Verification items for the finished model (mm, model axes). A direction names the side the tool comes from. Give positions to 0.01 mm unless a question says otherwise; leave off trailing zeros. Write each loop counter-clockwise with the first axis right and the second up, starting at its lowest first coordinate (ties: lowest second). Pieces come first, ordered by that corner, then holes. Notation, with made-up numbers: (-30.5, -7.75) - (7.5, -7.75) arc R23 ccw to (7.5, 5.25) - close; hole circle Ø8 at (47.5, 52.5). An arc over 180 degrees is marked (long way). Answer as a JSON object with one key per item and string values. Group by question number.
Item 1: Sectioned sample at B-B, the plane y = -47. Record the boundary of the cut face in (x, z).
Item 2: Sectioned sample at D-D, the plane x = -15.5. Record the boundary of the cut face in (y, z).
Item 3: Scan lines: line 1 along X through (y, z) = (-40.5, 19); line 2 along X through (y, z) = (12.5, 25.5); line 3 along Y through (x, z) = (-8, 12.5). Record each from-to range of solid material in increasing order. Write a range as [from, to].
Item 4: Tool access check on faces 1 (the face through (-105, -51.406, 20)), 2 (the face through (-109.732, -3, 20)), 3 (the face through (18, -56.406, 20)), 4 (the face through (-99.732, -10, 20)). Record the directions out of +Z, -Z, +X, -X, +Y, -Y that give a thin tool (end or side, any length) a straight path to the whole face; none if there is none.
Item 5: Sectioned sample at A-A, the plane y = -6. Record the boundary of the cut face in (x, z).
Item 6: Go/stop test with flat-tipped pins: pin 1 (2 mm diameter, centred on y = 3.5, z = 7, fed in from +X); pin 2 (1.5 mm diameter, centred on x = 41.5, z = 6, fed in from +Y); pin 3 (11 mm diameter, centred on x = -103.5, z = 28, fed in from -Y). Record where each tip stops, or that it passes through.
Item 7: Draft check along X on faces 5 (the face through (-33, -7, 0)), 6 (the face through (70.268, -53, 20)), 7 (the face through (-70, 33.594, 20)). Enter one of: +X half, -X half, draft (parallel to the pull), parting line (faces both ways), or undercut.
```python
from build123d import *

# Parameters (mm, degrees)
SKETCH_1_W      = 10
SKETCH_1_H      = 90
SKETCH_1_W_2    = 80
SKETCH_1_H_2    = 10
SKETCH_1_W_3    = 5
SKETCH_1_H_3    = 20
SKETCH_1_H_4    = 85
EXTRUDE_1_DEPTH = 40
FILLET_1_R      = 2.5


with BuildPart() as part:
    # 草圖1 → 填料-伸長1 (new body)
    with BuildSketch(Plane.XY):
        with Locations((-34.732391425, -11.40625)):
            Rectangle(SKETCH_1_W, SKETCH_1_H)
        Polygon((-29.732391425, -56.40625), (-39.732391425, -56.40625), (-39.732391425, -66.40625), (70.267608575, -66.40625), (70.267608575, -56.40625), (65.267608575, -56.40625), align=None)
        with Locations((-69.732391425, 38.59375)):
            Rectangle(SKETCH_1_W_2, SKETCH_1_H_2)
        with Locations((67.767608575, -46.40625)):
            Rectangle(SKETCH_1_W_3, SKETCH_1_H_3)
        with Locations((-104.732391425, -8.90625)):
            Rectangle(SKETCH_1_W, SKETCH_1_H_4)
    extrude(amount=EXTRUDE_1_DEPTH)

    # 圓角1
    fillet_1_edges = [part.edges().sort_by_distance(p)[0] for p in [
        (70.267608575, -36.40625, 20),
        (65.267608575, -36.40625, 20),
    ]]
    fillet(fillet_1_edges, radius=FILLET_1_R - 0.0001)  # a hair under: the kernel refuses the full size


solid = part.part
```
Geometry check:
{
 "1": {"outline": "(-109.73, 0) - (-99.73, 0) - (-99.73, 40) - (-109.73, 40) - close; (-39.73, 0) - (-29.73, 0) - (-29.73, 40) - (-39.73, 40) - close; (65.27, 0) - (70.27, 0) - (70.27, 40) - (65.27, 40) - close"},
 "2": {"outline": "(-66.41, 0) - (-56.41, 0) - (-56.41, 40) - (-66.41, 40) - close"},
 "3": {"line 1": "[-109.73, -99.73], [-39.73, -29.73], [65.27, 70.27]", "line 2": "[-109.73, -99.73], [-39.73, -29.73]", "line 3": "[-66.41, -56.41]"},
 "4": {"face 1": "+Z, -Z, -X, -Y", "face 2": "+Z, -Z, -X, +Y, -Y", "face 3": "+Z, -Z, +Y", "face 4": "+Z, -Z, -Y"},
 "5": {"outline": "(-109.73, 0) - (-99.73, 0) - (-99.73, 40) - (-109.73, 40) - close; (-39.73, 0) - (-29.73, 0) - (-29.73, 40) - (-39.73, 40) - close"},
 "6": {"pin 1": "x = -29.73", "pin 2": "y = -56.41", "pin 3": "y = -51.41"},
 "7": {"face 5": "draft", "face 6": "+X half", "face 7": "undercut"}
}
